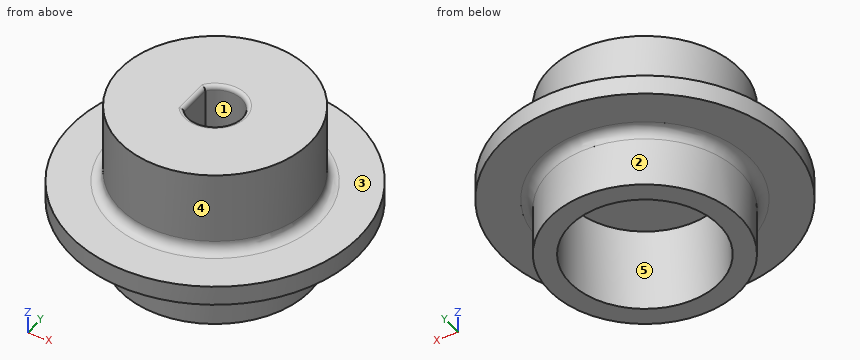
Autodesk Inventor part; units mm, degrees
ref_plane "YZ Plane" through (0, 0, 0) normal (1, 0, 0) x (0, 1, 0)
ref_plane "XZ Plane" through (0, 0, 0) normal (0, 1, 0) x (-1, 0, 0)
ref_plane "XY Plane" through (0, 0, 0) normal (0, 0, 1) x (1, 0, 0)
sketch "Sketch1" plane through (0, 0, 0) normal (0, 1, 0) x (-1, 0, 0)
  line L0 (0, 0) -> (2, 0)
  line L1 (2, 0) -> (2, 8.15)
  line L2 (2, 8.15) -> (0, 8.15)
  line L3 (0, 8.15) -> (0, 0)
  line L4 (0, 8.15) -> (9.25, 8.15)
  line L5 (9.25, 8.15) -> (9.25, 15.65)
  line L6 (9.25, 15.65) -> (0, 15.65)
  line L7 (0, 15.65) -> (0, 8.15)
  line L8 (0, 7.7) -> (-4.75, 7.7)
  line L9 (-4.75, 7.7) -> (-4.75, 5.8)
  line L10 (-4.75, 5.8) -> (0, 5.8)
  line L11 (0, 5.8) -> (0, 7.7)
  point P0 (0, 5.8)
  dimension "d1" = 7.25
  dimension "d2" = 2
  dimension "d3" = 7.5
  dimension "d4" = 8.15
  dimension "d10" = 14
  dimension "d12" = 1.9
  dimension "d13" = 7.95
revolve "Revolution1" add sketch "Sketch1" angle 360 about axis through (-9.25, 0, 8.15) along (0, 0, 1)
sketch "Sketch2" plane through (-9.25, 0, 15.65) normal (0, 0, 1) x (1, 0, 0)
  circle A0 centre (0, 0) radius 2.6
  line L0 (-2.0092, 1.6502) -> (-1.9908, -1.6724)
  circle A1 centre (0, 0) radius 9.25
  circle A2 centre (0, 0) radius 9.4
  point P0 (9.25, 0)
  dimension "d6" = 5.2
  dimension "d7" = 2
extrude "Extrusion1" cut sketch "Sketch2" against normal blind 10 contours A0 L0 picked at (-0.3829, 0.5768)
fillet "Fillet1" radius 1 2 edges at (-18.5, 0, 7.7) (-18.5, 0, 5.8)
fillet "Fillet2" radius 0.4 2 edges at (-6.65, 0.0144, 15.65) (-11.25, -0.0111, 15.65)
properties part number "Knob_adp"
Geometry check sheet. Reference: the model listing, model coordinates, mm. Face numbers are marked on the shaded views. A direction names the side the tool comes from. Give positions to 0.01 mm unless a question says otherwise; leave off trailing zeros. Loops run counter-clockwise (first coordinate to the right, second up) from the corner with the lowest first, then second, coordinate; pieces in that order, holes last.
(1) Section check D-D on x = 2.25. Record the cut outline in (y, z).
From the geometry:
outline: (-7.98, 5.8) - (7.98, 5.8) - (7.98, 7.7) - (-7.98, 7.7) - close
(2) Section check C-C on z = 2. Record the cut outline in (x, y), then the cut area to 3 significant figures.
From the geometry:
outline: circle Ø18.5 at (-9.25, 0); hole circle Ø14.5 at (-9.25, 0)
area: 104 mm2
(3) Set-up check for the marked faces 1 and 2: record each of +Z, -Z, +X, -X, +Y, -Y from which the full face is reachable in a straight line by a thin tool's end or side.
From the geometry:
face 1: +Z, -Z
face 2: -Z
(4) Thickness scan on L1, parallel to Y at x = -9.25, z = 2; L2, parallel to Y at x = -9.25, z = 11.5; L3, parallel to Z at x = -8.25, y = -12.5. Record the ranges inside material, lowest first.
From the geometry:
L1: y = -9.25 to -7.25, 7.25 to 9.25
L2: y = -9.25 to -2.6, 2.6 to 9.25
L3: z = 5.8 to 7.7
(5) Section check A-A on x = -9.25. Record the cut outline in (y, z), then the cut area to 3 significant figures.
From the geometry:
outline: (-14, 5.8) - (-10.25, 5.8) arc R1 cw to (-9.25, 4.8) - (-9.25, 0) - (-7.25, 0) - (-7.25, 8.15) - (-2.6, 8.15) - (-2.6, 15.25) arc R0.4 ccw to (-3, 15.65) - (-9.25, 15.65) - (-9.25, 8.7) arc R1 cw to (-10.25, 7.7) - (-14, 7.7) - close; (2.6, 8.15) - (7.25, 8.15) - (7.25, 0) - (9.25, 0) - (9.25, 4.8) arc R1 cw to (10.25, 5.8) - (14, 5.8) - (14, 7.7) - (10.25, 7.7) arc R1 cw to (9.25, 8.7) - (9.25, 15.65) - (3, 15.65) arc R0.4 ccw to (2.6, 15.25) - close
area: 151 mm2
(6) Section check B-B on z = 11. Record the cut outline in (x, y).
From the geometry:
outline: circle Ø18.5 at (-9.25, 0); hole (-11.26, 1.65) - (-11.24, -1.67) arc R2.6 ccw (long way) to start
(7) Release check for a two-part mould opening along Y. For the marked faces 3, 4 and 5 record: released by +Y, released by -Y, zero draft, split by the parting line, or undercut.
From the geometry:
face 3: zero draft
face 4: split by the parting line
face 5: undercut
(8) Depth check by flat-ended pin: pin 1 Ø8 at (x, z) = (-7, 10) entering from -Y; pin 2 Ø4 at (x, z) = (-11.5, 10.5) entering from -Y; pin 3 Ø13 at (x, y) = (-9.25, 0) entering from -Z; pin 4 Ø5 at (x, y) = (-1, 10) entering from +Z. Enter the tip coordinate at first touch or a pass-through.
From the geometry:
pin 1: stops at y = -14
pin 2: stops at y = -9.25
pin 3: stops at z = 8.15
pin 4: stops at z = 7.7
